Geometry: final body of the model. Coordinates: model frame, mm. Face numbers are marked on the shaded views. Coordinates: 2 decimals unless noted, no trailing zeros. Loops run counter-clockwise (first coordinate to the right, second up) from the corner with the lowest first, then second, coordinate; pieces in that order, holes last. Notation, with made-up numbers: (-40, -14) - (-3, -14) arc R32 ccw to (-3, 21) - close; hole circle Ø2 at (23, 1.25). An arc over 180 degrees is marked (long way). Return JSON: item names as keys, results as strings.
from build123d import *

# Parameters (mm, degrees)
SKETCH1_W                      = 223
SKETCH1_H                      = 153
BOSS_EXTRUDE2_DEPTH            = 8.5
SKETCH3_W                      = 154
SKETCH3_H                      = 93
CUT_EXTRUDE1_DEPTH             = 6
CUT_EXTRUDE3_REACH             = 137.487
CUT_EXTRUDE3_DIRECTION_2_REACH = 137.487
CHAMFER2_SIZE                  = 3


with BuildPart() as part:
    # Sketch1 → Boss-Extrude2 (new body)
    with BuildSketch(Plane(origin=(0, 0, 0), x_dir=(1, 0, 0), z_dir=(0, 1, 0))):
        Rectangle(SKETCH1_W, SKETCH1_H)
    extrude(amount=BOSS_EXTRUDE2_DEPTH)

    # Sketch3 → Cut-Extrude1 (cut)
    with BuildSketch(Plane(origin=(0, 8.5, 0), x_dir=(1, 0, 0), z_dir=(0, 1, 0))):
        Rectangle(SKETCH3_W, SKETCH3_H)
    extrude(amount=-CUT_EXTRUDE1_DEPTH, mode=Mode.SUBTRACT)

    # Cut-Extrude3: up to this face of the body (flat: up to its plane)
    cut_extrude3_end = Plane(part.part.faces().sort_by_distance((0, 4.25, -76.5))[0])
    # Sketch4 → Cut-Extrude3 (cut, up to the picked face)
    with BuildSketch(Plane.XY, mode=Mode.PRIVATE) as cut_extrude3_sk1:
        with BuildLine():
            Line((0, 8.5), (-111.5, 8.5))
            Line((-111.5, 8.5), (-111.5, 0))
            ThreePointArc((-111.5, 0), (-110.444247928, 2.707656577), (-107.834297931, 3.986006133))
            ThreePointArc((-107.834297931, 3.986006133), (-53.96436776, 7.371007599), (0, 8.5))
        make_face()
    cut_extrude3_tool1 = split(extrude(cut_extrude3_sk1.sketch, amount=-CUT_EXTRUDE3_REACH, mode=Mode.PRIVATE), bisect_by=cut_extrude3_end, keep=Keep.BOTH, mode=Mode.PRIVATE)
    # Sketch4 → Cut-Extrude3 (cut, up to the picked face)
    with BuildSketch(Plane.XY, mode=Mode.PRIVATE) as cut_extrude3_sk2:
        with BuildLine():
            Line((111.5, 8.5), (0, 8.5))
            ThreePointArc((0, 8.5), (53.96436776, 7.371007599), (107.834297931, 3.986006133))
            ThreePointArc((107.834297931, 3.986006133), (110.444247928, 2.707656577), (111.5, 0))
            Line((111.5, 0), (111.5, 8.5))
        make_face()
    cut_extrude3_tool2 = split(extrude(cut_extrude3_sk2.sketch, amount=-CUT_EXTRUDE3_REACH, mode=Mode.PRIVATE), bisect_by=cut_extrude3_end, keep=Keep.BOTH, mode=Mode.PRIVATE)
    add(cut_extrude3_tool1.solids().sort_by(Axis((-84.053137, 6.988854, 0), (0, 0, -1)))[0], mode=Mode.SUBTRACT)
    add(cut_extrude3_tool2.solids().sort_by(Axis((84.053137, 6.988854, 0), (0, 0, -1)))[0], mode=Mode.SUBTRACT)

    # Cut-Extrude3 direction 2: up to this face of the body (flat: up to its plane)
    cut_extrude3_direction_2_end = Plane(part.part.faces().sort_by_distance((0, 4.25, 76.5))[0])
    # Sketch4 → Cut-Extrude3 direction 2 (cut, up to the picked face)
    with BuildSketch(Plane.XY, mode=Mode.PRIVATE) as cut_extrude3_direction_2_sk1:
        with BuildLine():
            Line((0, 8.5), (-111.5, 8.5))
            Line((-111.5, 8.5), (-111.5, 0))
            ThreePointArc((-111.5, 0), (-110.444247928, 2.707656577), (-107.834297931, 3.986006133))
            ThreePointArc((-107.834297931, 3.986006133), (-53.96436776, 7.371007599), (0, 8.5))
        make_face()
    cut_extrude3_direction_2_tool1 = split(extrude(cut_extrude3_direction_2_sk1.sketch, amount=CUT_EXTRUDE3_DIRECTION_2_REACH, mode=Mode.PRIVATE), bisect_by=cut_extrude3_direction_2_end, keep=Keep.BOTH, mode=Mode.PRIVATE)
    # Sketch4 → Cut-Extrude3 direction 2 (cut, up to the picked face)
    with BuildSketch(Plane.XY, mode=Mode.PRIVATE) as cut_extrude3_direction_2_sk2:
        with BuildLine():
            Line((111.5, 8.5), (0, 8.5))
            ThreePointArc((0, 8.5), (53.96436776, 7.371007599), (107.834297931, 3.986006133))
            ThreePointArc((107.834297931, 3.986006133), (110.444247928, 2.707656577), (111.5, 0))
            Line((111.5, 0), (111.5, 8.5))
        make_face()
    cut_extrude3_direction_2_tool2 = split(extrude(cut_extrude3_direction_2_sk2.sketch, amount=CUT_EXTRUDE3_DIRECTION_2_REACH, mode=Mode.PRIVATE), bisect_by=cut_extrude3_direction_2_end, keep=Keep.BOTH, mode=Mode.PRIVATE)
    add(cut_extrude3_direction_2_tool1.solids().sort_by(Axis((-84.053137, 6.988854, 0), (0, 0, 1)))[0], mode=Mode.SUBTRACT)
    add(cut_extrude3_direction_2_tool2.solids().sort_by(Axis((84.053137, 6.988854, 0), (0, 0, 1)))[0], mode=Mode.SUBTRACT)

    # Chamfer2
    chamfer2_edges = [part.edges().sort_by_distance(p)[0] for p in [
        (77, 2.5, 0),
        (0, 2.5, 46.5),
        (-77, 2.5, 0),
        (0, 2.5, -46.5),
    ]]
    chamfer(chamfer2_edges, length=CHAMFER2_SIZE)


solid = part.part
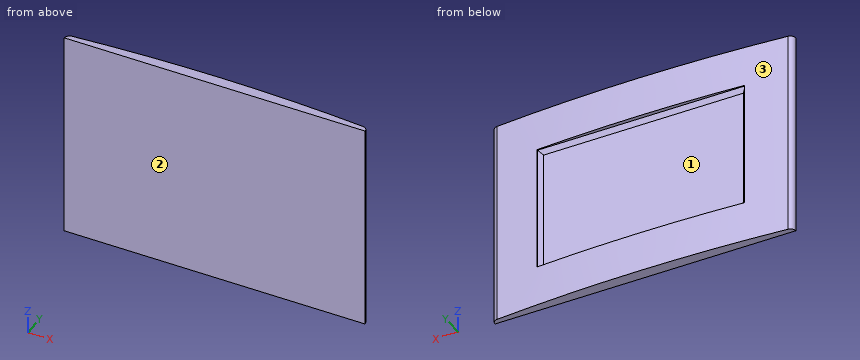
Item 1: Mould query, pull axis X, two halves, no side actions, for the marked faces 1, 2 and 3. Classes: +X half, -X half, draft (parallel to the pull), parting line (faces both ways), or undercut.
Worked out:
{"face 1": "undercut", "face 2": "draft", "face 3": "parting line"}
Item 2: Section query D-D, the plane x = -82.5. Return loops of the section in (y, z).
Worked out:
{"outline": "(0, -76.5) - (5.86, -76.5) - (5.86, 76.5) - (0, 76.5) - close"}
Item 3: Section query A-A, the plane z = -10.5. Return loops of the section in (x, y).
Worked out:
{"outline": "(-111.5, 0) - (111.5, 0) arc R4 ccw to (107.83, 3.99) arc R1290.28 ccw to (77, 6.2) - (77, 5.5) - (74, 2.5) - (-74, 2.5) - (-77, 5.5) - (-77, 6.2) arc R1290.28 ccw to (-107.83, 3.99) arc R4 ccw to start"}
Item 4: Section query B-B, the plane x = 43. Return loops of the section in (y, z).
Worked out:
{"outline": "(0, -76.5) - (7.78, -76.5) - (7.78, -46.5) - (5.5, -46.5) - (2.5, -43.5) - (2.5, 43.5) - (5.5, 46.5) - (7.78, 46.5) - (7.78, 76.5) - (0, 76.5) - close"}
Item 5: Ray query, probe 1 along Z at (x, y) = (-35, 6.5); probe 2 along X at (y, z) = (0.5, -61); probe 3 along Y at (x, z) = (-29.5, 2). Return the intervals inside material, ascending. Write a range as from..to.
Worked out:
{"probe 1": "-76.5..-46.5, 46.5..76.5", "probe 2": "-111.47..111.47", "probe 3": "0..2.5"}
Item 6: First-contact query: pin 1 Ø1 at (x, z) = (-77.5, -12.5) entering from +Y; pin 2 Ø4 at (x, z) = (29.5, 9) entering from +Y. Flat tips, straight axial feed; report the tip coordinate or a pass-through.
Worked out:
{"pin 1": "y = 6.2", "pin 2": "y = 2.5"}
Item 7: Section query C-C, the plane z = 61. Return loops of the section in (x, y).
Worked out:
{"outline": "(-111.5, 0) - (111.5, 0) arc R4 ccw to (107.83, 3.99) arc R1290.28 ccw to (-107.83, 3.99) arc R4 ccw to start"}
